from build123d import *

# Parameters (mm, degrees)
SKETCH_W                     = 10.5
SKETCH_H                     = 20
PAD_DEPTH                    = 1.6
SKETCH001_R                  = 0.245
POCKET_DEPTH                 = 46.891617
SKETCH001_LINEARPATTERN_2_R  = 0.245
POCKET_LINEARPATTERN_2_DEPTH = 46.891617
SKETCH001_LINEARPATTERN_3_R  = 0.245
POCKET_LINEARPATTERN_3_DEPTH = 46.891617
SKETCH001_LINEARPATTERN_4_R  = 0.245
POCKET_LINEARPATTERN_4_DEPTH = 46.891617
LINEARPATTERN001_COUNT       = 6
LINEARPATTERN001_PITCH       = 2.64


with BuildPart() as part:
    # Sketch → Pad (new body)
    with BuildSketch(Plane.XY):
        Rectangle(SKETCH_W, SKETCH_H)
    extrude(amount=PAD_DEPTH)

    # Sketch001 → Pocket (cut, through all)
    with BuildSketch(Plane.XY):
        with Locations((-3.75, 6.6)):
            Circle(SKETCH001_R)
    pocket = extrude(amount=POCKET_DEPTH, mode=Mode.SUBTRACT)

    # Sketch001 LinearPattern 2 → Pocket LinearPattern 2 (cut, through all)
    with BuildSketch(Plane(origin=(2.5, 0, 0), x_dir=(1, 0, 0), z_dir=(0, 0, 1))):
        with Locations((-3.75, 6.6)):
            Circle(SKETCH001_LINEARPATTERN_2_R)
    pocket_linearpattern_2 = extrude(amount=POCKET_LINEARPATTERN_2_DEPTH, mode=Mode.SUBTRACT)

    # Sketch001 LinearPattern 3 → Pocket LinearPattern 3 (cut, through all)
    with BuildSketch(Plane(origin=(5, 0, 0), x_dir=(1, 0, 0), z_dir=(0, 0, 1))):
        with Locations((-3.75, 6.6)):
            Circle(SKETCH001_LINEARPATTERN_3_R)
    pocket_linearpattern_3 = extrude(amount=POCKET_LINEARPATTERN_3_DEPTH, mode=Mode.SUBTRACT)

    # Sketch001 LinearPattern 4 → Pocket LinearPattern 4 (cut, through all)
    with BuildSketch(Plane(origin=(7.5, 0, 0), x_dir=(1, 0, 0), z_dir=(0, 0, 1))):
        with Locations((-3.75, 6.6)):
            Circle(SKETCH001_LINEARPATTERN_4_R)
    pocket_linearpattern_4 = extrude(amount=POCKET_LINEARPATTERN_4_DEPTH, mode=Mode.SUBTRACT)

    # LinearPattern001: Pocket, Pocket LinearPattern 2, Pocket LinearPattern 3, Pocket LinearPattern 4 ×6
    with Locations(*[(0, -i * LINEARPATTERN001_PITCH, 0) for i in range(1, LINEARPATTERN001_COUNT)]):
        add(pocket, mode=Mode.SUBTRACT)
        add(pocket_linearpattern_2, mode=Mode.SUBTRACT)
        add(pocket_linearpattern_3, mode=Mode.SUBTRACT)
        add(pocket_linearpattern_4, mode=Mode.SUBTRACT)


solid = part.part
Work out the finished part from the listing and answer in its coordinate system (mm). Coordinates: 2 decimals unless noted, no trailing zeros. Loops run counter-clockwise (first coordinate to the right, second up) from the corner with the lowest first, then second, coordinate; pieces in that order, holes last. Notation, with made-up numbers: M -1.5,34 L 27.5,34 A14 ccw 27.5,52 Z; hole C 5,17 d3. An arc over 180 degrees is marked long. Answer in a Markdown table with one row per item. Add a question column.
1. Find section C-C, the plane z = 1.1. State how many separate pieces and enclosed holes the cut face has, then the cut area to 3 significant figures.
2. Find section B-B, the plane y = -1.32. Write down the section's boundary in (x, z) (3 decimals).
3. A flat-ended cylindrical pin translates along its axis: P1, Ø2, axis at x = 3, y = 6.5, coming from the -Z side. Find the tip coordinate at first contact, or state that the pin passes through.
4. Consider L1, parallel to X at y = -1.32, z = 0.75 (3 decimals). Determine where the line is inside the solid, lowest interval first.
5. Find section A-A, the plane x = 3.75. Write down the section's boundary in (y, z) (3 decimals).
Reported:
| question | item | result |
|---|---|---|
| 1 | separate pieces | 1 |
| 1 | enclosed holes | 24 |
| 1 | area | 205 mm^2 |
| 2 | outline | M -5.25,0 L -3.995,0 L -3.995,1.6 L -5.25,1.6 Z; M -3.505,0 L -1.495,0 L -1.495,1.6 L -3.505,1.6 Z; M -1.005,0 L 1.005,0 L 1.005,1.6 L -1.005,1.6 Z; M 1.495,0 L 3.505,0 L 3.505,1.6 L 1.495,1.6 Z; M 3.995,0 L 5.25,0 L 5.25,1.6 L 3.995,1.6 Z |
| 3 | P1 | stops at z = 0 |
| 4 | L1 | x = -5.25 to -3.995, -3.505 to -1.495, -1.005 to 1.005, 1.495 to 3.505, 3.995 to 5.25 |
| 5 | outline | M -10,0 L -6.845,0 L -6.845,1.6 L -10,1.6 Z; M -6.355,0 L -4.205,0 L -4.205,1.6 L -6.355,1.6 Z; M -3.715,0 L -1.565,0 L -1.565,1.6 L -3.715,1.6 Z; M -1.075,0 L 1.075,0 L 1.075,1.6 L -1.075,1.6 Z; M 1.565,0 L 3.715,0 L 3.715,1.6 L 1.565,1.6 Z; M 4.205,0 L 6.355,0 L 6.355,1.6 L 4.205,1.6 Z; M 6.845,0 L 10,0 L 10,1.6 L 6.845,1.6 Z |
